Check sheet for the drawn part. Datum: minimum x, y, z corner. Units: mm. A direction names the side the tool comes from. Coordinates: 2 decimals unless noted, no trailing zeros. Write each loop counter-clockwise with the first axis right and the second up, starting at its lowest first coordinate (ties: lowest second). Pieces come first, ordered by that corner, then holes. Notation, with made-up numbers: M 52,-6.5 L 62,-6.5 A20 ccw 62,15.5 Z; hole C 35,75.25 d2. An arc over 180 degrees is marked long. Answer as a JSON object with one key per item and string values. Group by question number.
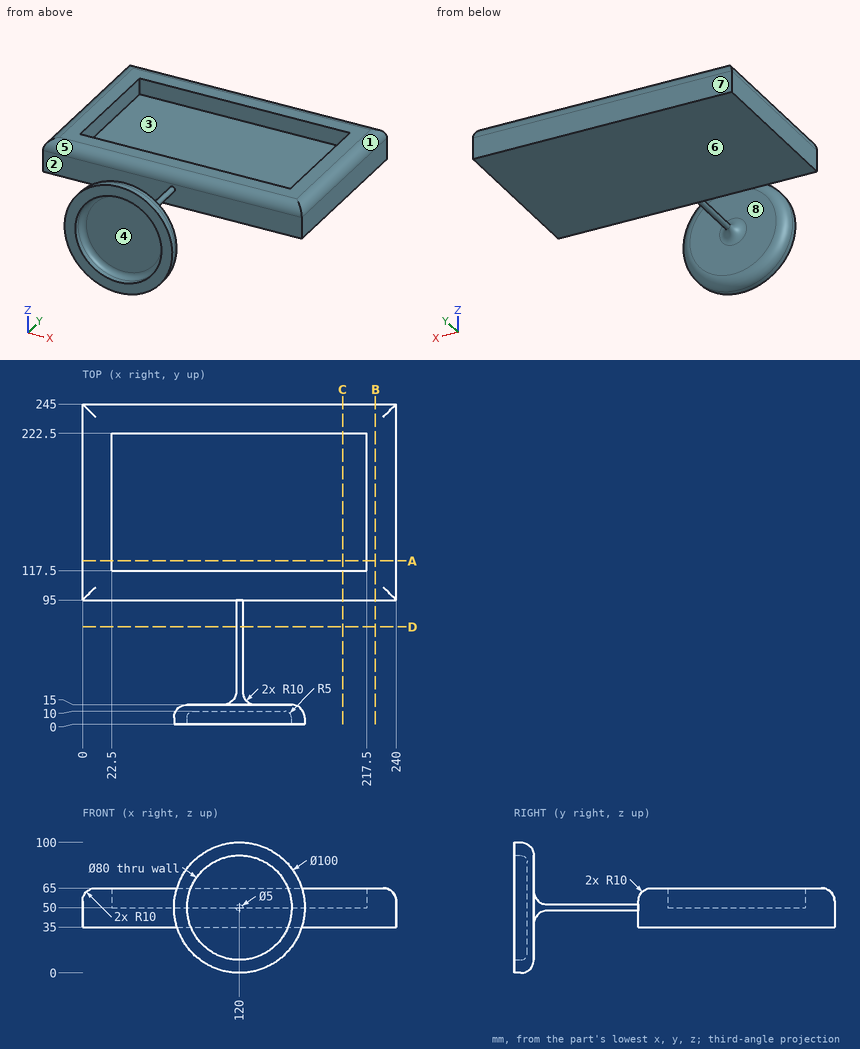
1) Section check B-B (x = 224). Record the cut outline in (y, z).
2) Go/stop test with flat-tipped pins: pin 1 Ø2 at (x, y) = (42.5, 113) entering from +Z; pin 2 Ø1.5 at (x, y) = (69, 219) entering from +Z. Record where each tip stops, or that it passes through.
3) Material ranges on probe 1 along X at (y, z) = (1.1, 50); probe 2 along Y at (x, z) = (208.5, 52); probe 3 along Y at (x, z) = (191.5, 38.5), recorded low to high. Write a range as [from, to].
4) Draft check along X on the marked faces 1, 2 and 3. Enter one of: +X half, -X half, draft (parallel to the pull), parting line (faces both ways), or undercut.
5) Section check C-C (x = 199). Record the cut outline in (y, z).
6) Section check A-A (y = 125). Record the cut outline in (x, z).
7) Set-up check for the marked faces 4, 5, 6, 7 and 8: record each of +Z, -Z, +X, -X, +Y, -Y from which the full face is reachable in a straight line by a thin tool's end or side.
8) Section check D-D (y = 74.5). Record the cut outline in (x, z), then the cut area to 3 significant figures.
Entries:
{
 "1": {"outline": "M 95,35 L 245,35 L 245,55 A10 ccw 235,65 L 105,65 A10 ccw 95,55 Z"},
 "2": {"pin 1": "z = 65", "pin 2": "z = 50"},
 "3": {"probe 1": "[70, 80], [160, 170]", "probe 2": "[95, 117.5], [222.5, 245]", "probe 3": "[95, 245]"},
 "4": {"face 1": "+X half", "face 2": "draft", "face 3": "undercut"},
 "5": {"outline": "M 95,35 L 245,35 L 245,55 A10 ccw 235,65 L 222.5,65 L 222.5,50 L 117.5,50 L 117.5,65 L 105,65 A10 ccw 95,55 Z"},
 "6": {"outline": "M 0,35 L 240,35 L 240,55 A10 ccw 230,65 L 217.5,65 L 217.5,50 L 22.5,50 L 22.5,65 L 10,65 A10 ccw 0,55 Z"},
 "7": {"face 4": "-Y", "face 5": "+Z, +X, -X", "face 6": "-Z, +X, -X, +Y", "face 7": "+Z, -Z, +X, -X, +Y", "face 8": "none"},
 "8": {"outline": "C 120,50 d5", "area": "19.6 mm^2"}
}
